The model under review builds one solid part; all positions refer to its coordinate system, in mm. A direction names the side the tool comes from. Round coordinates to 2 decimals unless told otherwise and drop trailing zeros. Loops run counter-clockwise (first coordinate to the right, second up) from the corner with the lowest first, then second, coordinate; pieces in that order, holes last. Notation, with made-up numbers: (-10, -1) -> (1, -1) arc R30 cw to (1, 34) -> close; hole circle Ø10 at (-1.5, 36). An arc over 180 degrees is marked (long way). Use a Markdown table: item, result. Add a question column.
1) Insertion check: pin 1 (3 mm diameter, centred on y = -4, z = 14.5, fed in from -X); pin 2 (4 mm diameter, centred on y = -22, z = 11, fed in from -X); pin 3 (1.8 mm diameter, centred on x = 17.5, z = 9, fed in from -Y). Each pin has a flat end and moves straight along its axis. Give the tip position at first contact, or say it passes through.
2) For faces 1 (the flat face through (24, -7, 9)), 2 (the flat face through (34, -7, 19)), 3 (the flat face through (21.994, -20, 10)), 4 (the flat face through (12, -9, 19)), 5 (the flat face through (20, -7, 11)), list the 3-axis set-ups (+Z, -Z, +X, -X, +Y, -Y) from which the entire face can be reached by the end or side of a thin tool; tool diameter is ignored.
3) Consider section B-B on y = -4.5. Give the boundary of the cut face in (x, z).
4) Mouldability with a two-part tool opening along X and no side actions: class faces 6 (the flat face through (12, 0, 2)), 7 (the cylindrical face through (5.01, -7.19, 2.03)), 8 (the flat face through (31.6, 5, 11)), 9 (the flat face through (0, -7, 21)) as released by +X, released by -X, zero draft, split by the parting line, or undercut.
5) Consider section C-C on x = 17. State how many separate pieces and enclosed holes the cut face has, plus the area to 3 significant figures.
6) Consider section D-D on z = 2.5. Give the boundary of the cut face in (x, y), plus the area to 3 significant figures.
7) Consider section A-A on y = -14. Give the boundary of the cut face in (x, z).
8) Wall thickness on probe 1 along Z at (x, y) = (6, -13.5); probe 2 along X at (y, z) = (-12, 12); probe 3 along Y at (x, z) = (21, 18.75): over which ranges is each line inside the solid? List them lowest first.
from build123d import *

# Parameters (mm, degrees)
F0_W     = 4
F0_H     = 15
F1_DEPTH = 15
F2_R     = 5
F3_DEPTH = 4.001
F4_R     = 2.25
F5_DEPTH = 4.001
F6_W     = 0.5
F6_H     = 8.5
F7_DEPTH = 10
F9_DEPTH = 7.6


with BuildPart() as f1:
    # F0 (on Front) → F1 (new body)
    with BuildSketch(Plane.XZ):
        Polygon((24, 0), (24, 4), (20, 4), (0, 4), (0, 0), align=None)
        with Locations((22, 11.5)):
            Rectangle(F0_W, F0_H)
        Polygon((20, 19), (24, 19), (44, 19), (44, 23), (0, 23), (0, 19), align=None)
    extrude(amount=F1_DEPTH)

    # F2 (on face) → F3 (cut, through all)
    with BuildSketch(Plane.XY.offset(4)):
        with Locations((10.0069084136, -7.405173449)):
            Circle(F2_R)
    extrude(amount=-F3_DEPTH, mode=Mode.SUBTRACT)

    # F4 (on face) → F5 (cut, through all)
    with BuildSketch(Plane(origin=(0, 0, 19), x_dir=(1, 0, 0), z_dir=(0, 0, -1))):
        with Locations((9.7508328035, 7.5500439852)):
            Circle(F4_R)
    extrude(amount=-F5_DEPTH, mode=Mode.SUBTRACT)

    # F6 (on face) → F7 (join)
    with BuildSketch(Plane.XZ.offset(15)):
        with Locations((21.7435011119, 10.0171177201)):
            Rectangle(F6_W, F6_H)
    extrude(amount=F7_DEPTH)

    # F8 (on face) → F9 (join, symmetric)
    with BuildSketch(Plane.YZ.offset(24)):
        with BuildLine():
            add(Edge.make_bspline(
                [(0, 15.6954114159), (6.5394724086, 14.608579241), (18.6393490716, 13.3520301619), (9.1807042924, 5.7328406438), (0, 5.3214114159)],
                knots=[0, 0, 0, 0, 0.4915313854, 1, 1, 1, 1], degree=3))
            Line((0, 15.6954114159), (0, 5.3214114159))
        make_face()
    extrude(amount=F9_DEPTH, both=True)


solid = f1.part
Result set:
| question | item | result |
|---|---|---|
| 1 | pin 1 | x = 20 |
| 1 | pin 2 | x = 21.49 |
| 1 | pin 3 | y = 0 |
| 2 | face 1 | -Z, +X, -Y |
| 2 | face 2 | -Z, +X, +Y, -Y |
| 2 | face 3 | +Z, -Z, +X, -Y |
| 2 | face 4 | -X, +Y, -Y |
| 2 | face 5 | -X, -Y |
| 3 | outline | (0, 0) -> (5.94, 0) -> (5.94, 4) -> (0, 4) -> close; (0, 19) -> (20, 19) -> (20, 4) -> (14.08, 4) -> (14.08, 0) -> (24, 0) -> (24, 19) -> (44, 19) -> (44, 23) -> (0, 23) -> close |
| 4 | face 6 | zero draft |
| 4 | face 7 | undercut |
| 4 | face 8 | released by +X |
| 4 | face 9 | released by -X |
| 5 | separate pieces | 3 |
| 5 | enclosed holes | 0 |
| 5 | area | 221 mm2 |
| 6 | outline | (0, -15) -> (24, -15) -> (24, 0) -> (0, 0) -> close; hole circle Ø10 at (10.01, -7.41) |
| 6 | area | 281 mm2 |
| 7 | outline | (0, 0) -> (24, 0) -> (24, 19) -> (44, 19) -> (44, 23) -> (0, 23) -> (0, 19) -> (20, 19) -> (20, 4) -> (0, 4) -> close |
| 8 | probe 1 | 0 to 4, 19 to 23 |
| 8 | probe 2 | 20 to 24 |
| 8 | probe 3 | -15 to 0 |
